CAD build for the part. Positions are in the model's coordinates, mm. Face numbers are marked on the shaded views. Round coordinates to 2 decimals unless told otherwise and drop trailing zeros. Write each loop counter-clockwise with the first axis right and the second up, starting at its lowest first coordinate (ties: lowest second). Pieces come first, ordered by that corner, then holes. Notation, with made-up numbers: (11.5, -21) - (68.5, -21) arc R30 cw to (68.5, 3) - close; hole circle Ø3 at (46, -31). An arc over 180 degrees is marked (long way). Use one line per item in the form item = value. Start each with the question number.
Item 1: Pull direction Z, two halves, no side cores. Call the marked faces 1, 2 and 3: +Z half, -Z half, draft (parallel to the pull), parting line (faces both ways), or undercut.
Item 2: Band-saw the part on A-A, the plane z = -5.75. List the corners of the cut face in (x, y).
Item 3: Band-saw the part on B-B, the plane x = -1.75. List the corners of the cut face in (y, z).
Item 4: Drill centre lines: L1, parallel to X at y = 1.2, z = -5; L2, parallel to X at y = 1.5, z = -5.5; L3, parallel to Z at x = -5.25, y = 1.8. Where is each one in solid material? Low to high.
Item 5: Band-saw the part on C-C, the plane y = 1.55. List the corners of the cut face in (x, z).
Item 6: Band-saw the part on D-D, the plane x = -0.25. List the corners of the cut face in (y, z), and give its area (3 significant figures).
Item 7: Pin check, flat tips, straight feed: pin 1 (1 mm diameter, centred on y = 2.5, z = -1, fed in from -X); pin 2 (1 mm diameter, centred on x = -1, y = 0.5, fed in from -Z); pin 3 (1 mm diameter, centred on y = 2, z = -6, fed in from -X). Stop position of each tip, or through.
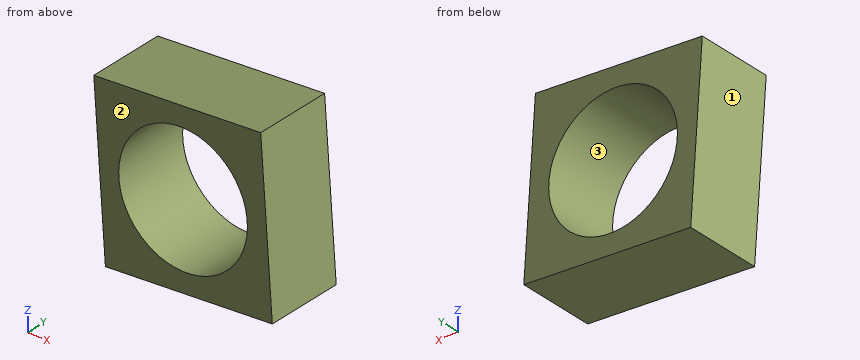
from build123d import *

# Parameters (mm, degrees)
BOSS_EXTRUDE1_DEPTH = 3
SKETCH3_R           = 2.5
CUT_EXTRUDE1_DEPTH  = 3


with BuildPart() as part:
    # Sketch2 → Boss-Extrude1 (new body)
    with BuildSketch(Plane(origin=(0, 0, 0), x_dir=(1, 0, 0), z_dir=(0, 1, 0))):
        Polygon((0, 0), (0.450772745, 6.484350695), (-6.03357795, 6.93512344), (-6.484350695, 0.450772745), align=None)
    extrude(amount=BOSS_EXTRUDE1_DEPTH)

    # Sketch3 → Cut-Extrude1 (cut)
    with BuildSketch(Plane(origin=(0, 3, 0), x_dir=(1, 0, 0), z_dir=(0, 1, 0))):
        with Locations(Location((-3.016788975, 3.46756172, 0), (0, 0, 270))):
            Circle(SKETCH3_R)
    extrude(amount=-CUT_EXTRUDE1_DEPTH, mode=Mode.SUBTRACT)


solid = part.part
Determined:
q1.face_1 = -Z half
q1.face_2 = draft
q1.face_3 = undercut
q2.outline = (-6.12, 0) - (-4.04, 0) - (-4.04, 3) - (-6.12, 3) - close; (-2, 0) - (0.4, 0) - (0.4, 3) - (-2, 3) - close
q3.outline = (0, -6.64) - (3, -6.64) - (3, -5.62) - (0, -5.62) - close; (0, -1.31) - (3, -1.31) - (3, -0.12) - (0, -0.12) - close
q4.L1 = -6.17 to -4.99, -1.04 to 0.35
q4.L2 = -6.13 to -4.47, -1.56 to 0.38
q4.L3 = -6.88 to -4.59, -2.34 to -0.36
q5.outline = (-6.48, -0.45) - (-6.03, -6.94) - (0.45, -6.48) - (0, 0) - close; hole circle Ø5 at (-3.02, -3.47)
q6.outline = (0, -6.53) - (3, -6.53) - (3, -0.02) - (0, -0.02) - close
q6.area = 19.5 mm²
q7.pin_1 = -6.48
q7.pin_2 = -6.62
q7.pin_3 = -6.13
